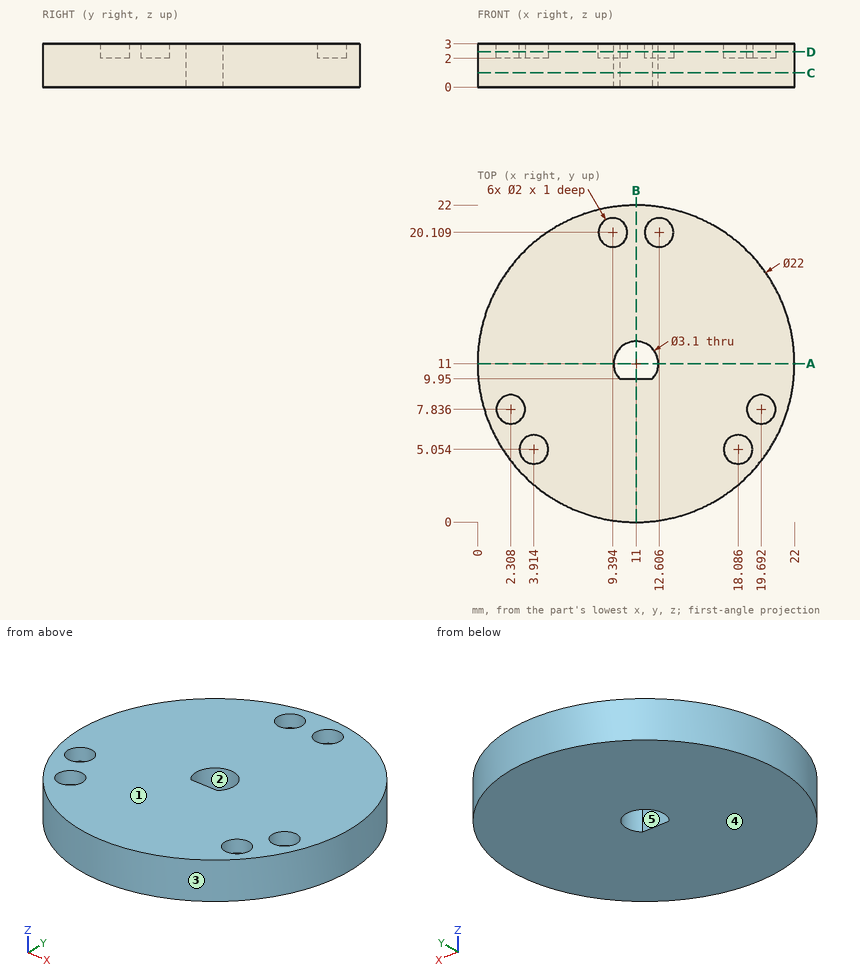
Here's the drawing with two shaded views (mm, measured from the low corner). I have some questions. A direction names the side the tool comes from. Round coordinates to 2 decimals unless told otherwise and drop trailing zeros. Loops run counter-clockwise (first coordinate to the right, second up) from the corner with the lowest first, then second, coordinate; pieces in that order, holes last.
1. Suppose I cut it at D-D, the plane z = 2.45. Give the number of separate pieces and of enclosed holes in the cut face.
Answers:
separate pieces: 1
enclosed holes: 7
2. Suppose I cut it at C-C, the plane z = 1. Please give me the cut outline in (x, y).
Answers:
outline: circle Ø22 at (11, 11); hole (9.86, 9.95) - (12.14, 9.95) arc R1.55 ccw (long way) to start
3. Will these pins go through, and if not, where does the flat tip stop? pin 1 (1.6 mm diameter, centred on x = 3.91, y = 5.05, fed in from +Z); pin 2 (1.5 mm diameter, centred on x = 12.5, z = 1, fed in from -Y) (1 decimal).
Answers:
pin 1: stops at z = 2
pin 2: stops at y = 0
4. Suppose I cut it at A-A, the plane y = 11. Please give me the cut outline in (x, z).
Answers:
outline: (0, 0) - (9.45, 0) - (9.45, 3) - (0, 3) - close; (12.55, 0) - (22, 0) - (22, 3) - (12.55, 3) - close
5. Thinking about a two-plate mould opening in X: for the marked faces 1, 2 and 3, which applies, released by +X, released by -X, zero draft, split by the parting line, or undercut?
Answers:
face 1: zero draft
face 2: undercut
face 3: split by the parting line
6. Suppose I cut it at B-B, the plane x = 11. Please give me the cut outline in (y, z), and give its area (3 significant figures).
Answers:
outline: (0, 0) - (9.95, 0) - (9.95, 3) - (0, 3) - close; (12.55, 0) - (22, 0) - (22, 3) - (12.55, 3) - close
area: 58.2 mm2
7. If I drill on probe 1 along Y at (x, z) = (11, 1.35); probe 2 along Y at (x, z) = (2.75, 0.3) (1 decimal); probe 3 along Z at (x, y) = (19.25, 7.75), over which ranges is the centre line in solid material (lowest first)?
Answers:
probe 1: y = 0 to 9.95, 12.55 to 22
probe 2: y = 3.7 to 18.3
probe 3: z = 0 to 2
8. For the marked faces 4 and 5, which set-ups out of +Z, -Z, +X, -X, +Y, -Y let a thin tool reach every point of the face, with its end or its side?
Answers:
face 4: -Z, +X, -X, +Y, -Y
face 5: +Z, -Z
